Design review of the part built by this model. Coordinates are the model's own, in mm. A direction names the side the tool comes from. Coordinates: 2 decimals unless noted, no trailing zeros. Loops run counter-clockwise (first coordinate to the right, second up) from the corner with the lowest first, then second, coordinate; pieces in that order, holes last.
Q1. Add section B-B on x = -33.5. Give the boundary of the cut face in (y, z), and give its area (3 significant figures).
Q2. For P1, Ø7.5, axis at x = 127, z = 0, coming from the +Y side, flat-tipped, find the tip position at first contact; note if it passes through.
Q3. Wall thickness on probe 1 along Z at (x, y) = (-139, 2.5); probe 2 along Z at (x, y) = (-26.5, 9.25): over which ranges is each line inside the solid? List them lowest first.
Q4. Machinability: for faces 1 (the face through (3, 12.7, 0)), 2 (the face through (3, -11.112, 0)), 3 (the face through (-119.13, 11.92, -1.03)), which of the approach directions +Z, -Z, +X, -X, +Y, -Y give a long, thin tool a straight path to every point of the face, cutting with its end or side? Answer none if there is none.
Q5. Add section A-A on y = 4.5. Give the boundary of the cut face in (x, z), and give its area (3 significant figures).
Q6. Draft analysis for pull direction X (two halves, no side actions). For faces 4 (the face through (3, 0, 12.7)), 5 (the face through (241.3, 1, 11.3)), 6 (the face through (134.87, 11.92, -1.03)), state which applies: released by +X, released by -X, zero draft, split by the parting line, or undercut.
```python
from build123d import *

# Parameters (mm, degrees)
SKETCH1_W           = 25.4
SKETCH1_H           = 25.4
SKETCH1_W_2         = 22.225
SKETCH1_H_2         = 22.225
BOSS_EXTRUDE1_DEPTH = 241.3
FILLET1_R           = 2.54
CUT_EXTRUDE1_REACH  = 244.965
SKETCH2_R           = 3.175
CUT_EXTRUDE2_REACH  = 244.965
SKETCH3_R           = 7.9375
CUT_EXTRUDE3_REACH  = 244.965
SKETCH4_R           = 3.175


with BuildPart() as part:
    # Sketch1 → Boss-Extrude1 (new, symmetric)
    with BuildSketch(Plane(origin=(0, 0, 0), x_dir=(0, 0, -1), z_dir=(1, 0, 0))):
        Rectangle(SKETCH1_W, SKETCH1_H)
        Rectangle(SKETCH1_W_2, SKETCH1_H_2, mode=Mode.SUBTRACT)
    extrude(amount=BOSS_EXTRUDE1_DEPTH, both=True)

    # Fillet1
    fillet1_edges = [part.edges().sort_by_distance(p)[0] for p in [
        (0, -11.1125, -11.1125),
        (0, 11.1125, -11.1125),
        (0, 11.1125, 11.1125),
        (0, -11.1125, 11.1125),
        (0, -12.7, -12.7),
        (0, -12.7, 12.7),
        (0, 12.7, 12.7),
        (0, 12.7, -12.7),
    ]]
    fillet(fillet1_edges, radius=FILLET1_R)

    # Sketch2 → Cut-Extrude1 (cut, up to next)
    with BuildSketch(Plane(origin=(0, -12.7, 0), x_dir=(1, 0, 0), z_dir=(0, 1, 0)), mode=Mode.PRIVATE) as cut_extrude1_sk1:
        with Locations(Location((127, 0, 0), (0, 0, 90))):
            Circle(SKETCH2_R)
    cut_extrude1_tool1 = extrude(cut_extrude1_sk1.sketch, amount=CUT_EXTRUDE1_REACH, mode=Mode.PRIVATE) & part.part
    # Sketch2 → Cut-Extrude1 (cut, up to next)
    with BuildSketch(Plane(origin=(0, -12.7, 0), x_dir=(1, 0, 0), z_dir=(0, 1, 0)), mode=Mode.PRIVATE) as cut_extrude1_sk2:
        with Locations(Location((-127, 0, 0), (0, 0, 90))):
            Circle(SKETCH2_R)
    cut_extrude1_tool2 = extrude(cut_extrude1_sk2.sketch, amount=CUT_EXTRUDE1_REACH, mode=Mode.PRIVATE) & part.part
    add(cut_extrude1_tool1.solids().sort_by_distance((127, -12.7, 0))[0], mode=Mode.SUBTRACT)
    add(cut_extrude1_tool2.solids().sort_by_distance((-127, -12.7, 0))[0], mode=Mode.SUBTRACT)

    # Sketch3 → Cut-Extrude2 (cut, up to next)
    with BuildSketch(Plane(origin=(0, 12.7, 0), x_dir=(1, 0, 0), z_dir=(0, 1, 0)), mode=Mode.PRIVATE) as cut_extrude2_sk1:
        with Locations(Location((-127, 0, 0), (0, 0, 270))):
            Circle(SKETCH3_R)
    cut_extrude2_tool1 = extrude(cut_extrude2_sk1.sketch, amount=-CUT_EXTRUDE2_REACH, mode=Mode.PRIVATE) & part.part
    # Sketch3 → Cut-Extrude2 (cut, up to next)
    with BuildSketch(Plane(origin=(0, 12.7, 0), x_dir=(1, 0, 0), z_dir=(0, 1, 0)), mode=Mode.PRIVATE) as cut_extrude2_sk2:
        with Locations(Location((127, 0, 0), (0, 0, 270))):
            Circle(SKETCH3_R)
    cut_extrude2_tool2 = extrude(cut_extrude2_sk2.sketch, amount=-CUT_EXTRUDE2_REACH, mode=Mode.PRIVATE) & part.part
    add(cut_extrude2_tool1.solids().sort_by_distance((-127, 12.7, 0))[0], mode=Mode.SUBTRACT)
    add(cut_extrude2_tool2.solids().sort_by_distance((127, 12.7, 0))[0], mode=Mode.SUBTRACT)

    # Cut-Extrude3: up to this face of the body (flat: up to its plane)
    cut_extrude3_end = Plane(part.part.faces().sort_by_distance((0, -12.7, 0))[0])
    # Sketch4 → Cut-Extrude3 (cut, up to the picked face)
    with BuildSketch(Plane(origin=(0, 12.7, 0), x_dir=(1, 0, 0), z_dir=(0, 1, 0)), mode=Mode.PRIVATE) as cut_extrude3_sk1:
        with Locations(Location((-228.6, 0, 0), (0, 0, 270))):
            Circle(SKETCH4_R)
    cut_extrude3_tool1 = split(extrude(cut_extrude3_sk1.sketch, amount=-CUT_EXTRUDE3_REACH, mode=Mode.PRIVATE), bisect_by=cut_extrude3_end, keep=Keep.BOTH, mode=Mode.PRIVATE)
    # Sketch4 → Cut-Extrude3 (cut, up to the picked face)
    with BuildSketch(Plane(origin=(0, 12.7, 0), x_dir=(1, 0, 0), z_dir=(0, 1, 0)), mode=Mode.PRIVATE) as cut_extrude3_sk2:
        with Locations(Location((-212.725, 0, 0), (0, 0, 270))):
            Circle(SKETCH4_R)
    cut_extrude3_tool2 = split(extrude(cut_extrude3_sk2.sketch, amount=-CUT_EXTRUDE3_REACH, mode=Mode.PRIVATE), bisect_by=cut_extrude3_end, keep=Keep.BOTH, mode=Mode.PRIVATE)
    cut_extrude3_1 = cut_extrude3_tool1.solids().sort_by(Axis((-228.6, 12.7, 0), (0, -1, 0)))[0]
    add(cut_extrude3_1, mode=Mode.SUBTRACT)
    cut_extrude3_2 = cut_extrude3_tool2.solids().sort_by(Axis((-212.725, 12.7, 0), (0, -1, 0)))[0]
    add(cut_extrude3_2, mode=Mode.SUBTRACT)
    cut_extrude3 = cut_extrude3_1 + cut_extrude3_2  # Cut-Extrude3 as one shape, for the pattern or mirror that repeats it

    # Mirror1: Cut-Extrude3 across plane
    add(cut_extrude3.mirror(Plane(origin=(0, 0, 0), x_dir=(0, 0, 1), z_dir=(1, 0, 0))), mode=Mode.SUBTRACT)


solid = part.part
```
Entries:
1. outline: (-12.7, -10.16) arc R2.54 ccw to (-10.16, -12.7) - (10.16, -12.7) arc R2.54 ccw to (12.7, -10.16) - (12.7, 10.16) arc R2.54 ccw to (10.16, 12.7) - (-10.16, 12.7) arc R2.54 ccw to (-12.7, 10.16) - close; hole (-11.11, -8.57) arc R2.54 ccw to (-8.57, -11.11) - (8.57, -11.11) arc R2.54 ccw to (11.11, -8.57) - (11.11, 8.57) arc R2.54 ccw to (8.57, 11.11) - (-8.57, 11.11) arc R2.54 ccw to (-11.11, 8.57) - close
1. area: 151 mm2
2. P1: stops at y = -11.11
3. probe 1: z = -12.7 to -11.11, 11.11 to 12.7
3. probe 2: z = -12.7 to -11.02, 11.02 to 12.7
4. face 1: +Z, -Z, +X, -X, +Y
4. face 2: +X, -X
4. face 3: +Y
5. outline: (-241.3, -12.7) - (241.3, -12.7) - (241.3, -11.11) - (-241.3, -11.11) - close; (-241.3, 11.11) - (241.3, 11.11) - (241.3, 12.7) - (-241.3, 12.7) - close
5. area: 1,530 mm2
6. face 4: zero draft
6. face 5: released by +X
6. face 6: undercut
